Here's the drawing with two shaded views (mm, measured from the low corner). I have some questions. A direction names the side the tool comes from. Round coordinates to 2 decimals unless told otherwise and drop trailing zeros. Loops run counter-clockwise (first coordinate to the right, second up) from the corner with the lowest first, then second, coordinate; pieces in that order, holes last. Notation, with made-up numbers: M 78,28 L 103,28 A9 ccw 103,45 Z; hole C -30.5,-6.75 d9. An arc over 180 degrees is marked long. Answer as a JSON object with one key per item and string values.
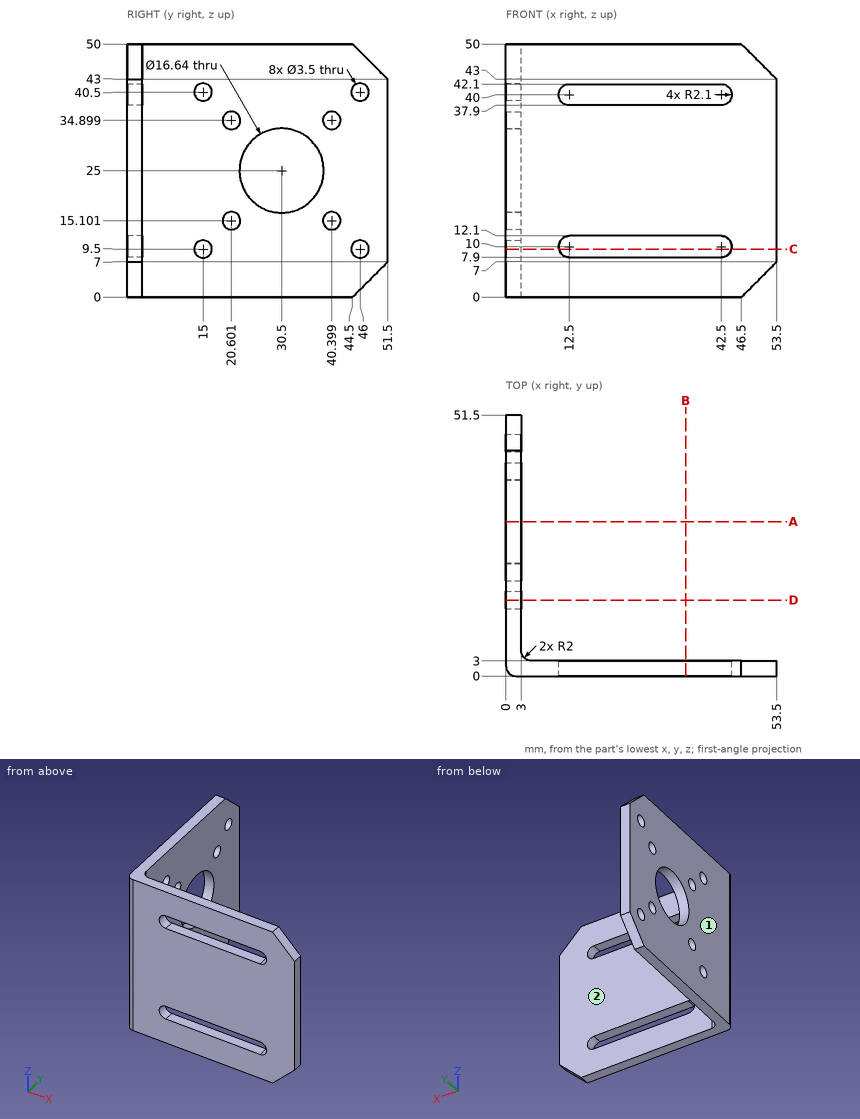
Item 1: If I drill on L1, parallel to Y at x = 47.5, z = 14; L2, parallel to Y at x = 1.6, z = 9.5, over which ranges is the centre line in solid material (lowest first)? Write a range as from..to.
Solution:
{"L1": "y = 0..3", "L2": "y = 0.04..13.25, 16.75..44.25, 47.75..51.5"}
Item 2: I want a section at C-C on z = 9.5. List the corners of the cut face in (x, y) for me.
Solution:
{"outline": "M 0,2 A2 ccw 2,0 L 10.46,0 L 10.46,3 L 5,3 A2 cw 3,5 L 3,13.25 L 0,13.25 Z; M 0,16.75 L 3,16.75 L 3,44.25 L 0,44.25 Z; M 0,47.75 L 3,47.75 L 3,51.5 L 0,51.5 Z; M 44.54,0 L 53.5,0 L 53.5,3 L 44.54,3 Z"}
Item 3: I want a section at B-B on x = 35.5. List the corners of the cut face in (y, z) for me, plus the area to 3 significant figures.
Solution:
{"outline": "M 0,0 L 3,0 L 3,7.9 L 0,7.9 Z; M 0,12.1 L 3,12.1 L 3,37.9 L 0,37.9 Z; M 0,42.1 L 3,42.1 L 3,50 L 0,50 Z", "area": "125 mm2"}
Item 4: I want a section at D-D on y = 15. List the corners of the cut face in (x, z) for me.
Solution:
{"outline": "M 0,0 L 3,0 L 3,7.75 L 0,7.75 Z; M 0,11.25 L 3,11.25 L 3,38.75 L 0,38.75 Z; M 0,42.25 L 3,42.25 L 3,50 L 0,50 Z"}
Item 5: I want a section at A-A on y = 30.5. List the corners of the cut face in (x, z) for me.
Solution:
{"outline": "M 0,0 L 3,0 L 3,16.68 L 0,16.68 Z; M 0,33.32 L 3,33.32 L 3,50 L 0,50 Z"}
Item 6: For the marked faces 1 and 2, which set-ups out of +Z, -Z, +X, -X, +Y, -Y let a thin tool reach every point of the face, with its end or its side?
Solution:
{"face 1": "+Z, -Z, -X, +Y, -Y", "face 2": "+Z, -Z, +X, +Y"}
Item 7: For P1, Ø4, axis at y = 46, z = 9.5, coming from the +X side; P2, Ø3, axis at y = 15, z = 9.5, coming from the -X side; P3, Ø8, axis at x = 13.5, z = 7.5, coming from the +Y side; P4, Ø12, axis at y = 10, z = 5.5, coming from the +X side, each with a flat end and sliding along its axis, tell me the tip position at first contact or that it passes through.
Solution:
{"P1": "stops at x = 3", "P2": "passes through", "P3": "stops at y = 3", "P4": "stops at x = 3.27"}
